Design review of the part built by this model. Coordinates are the model's own, in mm. Give positions to 0.01 mm unless a question says otherwise; leave off trailing zeros. Write each loop counter-clockwise with the first axis right and the second up, starting at its lowest first coordinate (ties: lowest second). Pieces come first, ordered by that corner, then holes. Notation, with made-up numbers: M -27.5,47 L 24.5,47 A32 cw 24.5,84 Z; hole C -24,19.5 d6. An arc over 180 degrees is marked long. Answer in a Markdown table with one row per item.
```python
from build123d import *

# Parameters (mm, degrees)
SKETCH3_R           = 50.7685
SKETCH3_R_2         = 3.785
SKETCH3_R_3         = 0.925
SKETCH3_R_4         = 2.275
SKETCH3_W           = 12.7001
SKETCH3_H           = 9.9
SKETCH3_W_2         = 6.25
SKETCH3_H_2         = 3
SKETCH3_W_3         = 20.5
BOSS_EXTRUDE7_DEPTH = 5


with BuildPart() as part:
    # Sketch3 → Boss-Extrude7 (new body)
    with BuildSketch(Plane.XY):
        with Locations((60.71181161, 107.410494733)):
            Circle(SKETCH3_R)
        with Locations((60.71181161, 107.410494733)):
            Circle(SKETCH3_R_2, mode=Mode.SUBTRACT)
        with Locations((65.96181161, 102.060494733)):
            Circle(SKETCH3_R_3, mode=Mode.SUBTRACT)
        with Locations((38.0489, 92.578417091)):
            Circle(SKETCH3_R_4, mode=Mode.SUBTRACT)
        with Locations((84.0509, 92.578417091)):
            Circle(SKETCH3_R_4, mode=Mode.SUBTRACT)
        with Locations((84.0509, 122.242572375)):
            Circle(SKETCH3_R_4, mode=Mode.SUBTRACT)
        with Locations((38.0489, 122.242572375)):
            Circle(SKETCH3_R_4, mode=Mode.SUBTRACT)
        with Locations((55.46181161, 102.060494733)):
            Circle(SKETCH3_R_3, mode=Mode.SUBTRACT)
        with Locations((65.96181161, 112.760494733)):
            Circle(SKETCH3_R_3, mode=Mode.SUBTRACT)
        with Locations((55.46181161, 112.760494733)):
            Circle(SKETCH3_R_3, mode=Mode.SUBTRACT)
        with Locations((34.28955, 107.410494733)):
            Rectangle(SKETCH3_W, SKETCH3_H, mode=Mode.SUBTRACT)
        with Locations((28.0289, 92.578417091)):
            Rectangle(SKETCH3_W_2, SKETCH3_H_2, mode=Mode.SUBTRACT)
        with Locations((66.1289, 92.578417091)):
            Rectangle(SKETCH3_W_3, SKETCH3_H_2, mode=Mode.SUBTRACT)
        with Locations((94.0689, 92.578417091)):
            Rectangle(SKETCH3_W_2, SKETCH3_H_2, mode=Mode.SUBTRACT)
        with Locations((28.0289, 122.242572375)):
            Rectangle(SKETCH3_W_2, SKETCH3_H_2, mode=Mode.SUBTRACT)
        with Locations((66.1289, 122.242572375)):
            Rectangle(SKETCH3_W_3, SKETCH3_H_2, mode=Mode.SUBTRACT)
        with Locations((94.0689, 122.242572375)):
            Rectangle(SKETCH3_W_2, SKETCH3_H_2, mode=Mode.SUBTRACT)
        with Locations((87.13407322, 107.410494733)):
            Rectangle(SKETCH3_W, SKETCH3_H, mode=Mode.SUBTRACT)
    extrude(amount=BOSS_EXTRUDE7_DEPTH)


solid = part.part
```
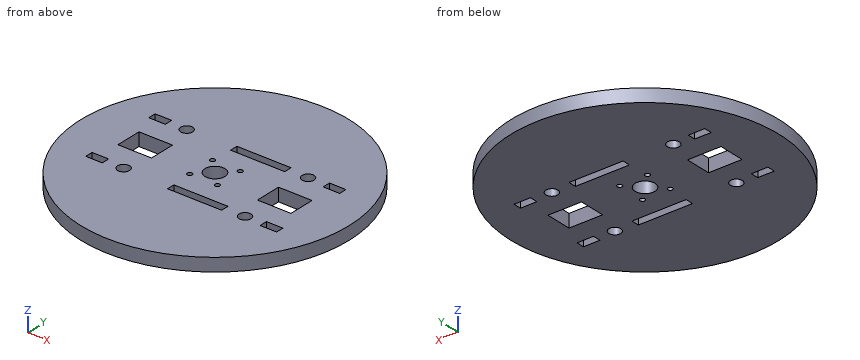
1) Add section C-C (x = 99). Write out the cut boundary in (y, z).
Geometry says:
| item | result |
|---|---|
| outline | M 74.07,0 L 140.75,0 L 140.75,5 L 74.07,5 Z |
2) Add section A-A (x = 74.5). Write out the cut boundary in (y, z), and give its area (3 significant figures).
Geometry says:
| item | result |
|---|---|
| outline | M 58.55,0 L 91.08,0 L 91.08,5 L 58.55,5 Z; M 94.08,0 L 120.74,0 L 120.74,5 L 94.08,5 Z; M 123.74,0 L 156.27,0 L 156.27,5 L 123.74,5 Z |
| area | 459 mm^2 |
3) Add section D-D (z = 3.65). Count the separate pieces of the cut face and the enclosed holes in it, and give its area (3 significant figures).
Geometry says:
| item | result |
|---|---|
| separate pieces | 1 |
| enclosed holes | 17 |
| area | 7,530 mm^2 |
4) Add section B-B (y = 78). Write out the cut boundary in (x, z).
Geometry says:
| item | result |
|---|---|
| outline | M 19.33,0 L 102.09,0 L 102.09,5 L 19.33,5 Z |
5) To check wall thickness, follow probe 1 along Y at (x, z) = (96.5, 2.3); probe 2 along Y at (x, z) = (85.5, 4.45); probe 3 along X at (y, z) = (103.5, 2.05). State the ranges of each line that lie inside material, in increasing order. Write a range as [from, to].
Geometry says:
| item | result |
|---|---|
| probe 1 | [71.4, 91.08], [94.08, 120.74], [123.74, 143.42] |
| probe 2 | [63.1, 90.82], [94.33, 102.46], [112.36, 120.49], [124, 151.72] |
| probe 3 | [10.09, 27.94], [40.64, 80.78], [93.48, 111.33] |
6) Insertion check: P1, Ø7.5, axis at x = 84.05, y = 92.58, coming from the +Z side; P2, Ø1.1, axis at x = 65.96, y = 112.76, coming from the -Z side; P3, Ø1, axis at x = 42.5, z = 3.5, coming from the +Y side; P4, Ø2.5, axis at x = 93.5, z = 3, coming from the -Y side. Each pin has a flat end and moves straight along its axis. Give the tip position at first contact, or say it passes through.
Geometry says:
| item | result |
|---|---|
| P1 | z = 5 |
| P2 | through |
| P3 | y = 154.99 |
| P4 | y = 67.63 |
